Could you check a few things on this drawing? It's one solid part, dimensions in mm from its lowest x, y, z. Coordinates: 2 decimals unless noted, no trailing zeros. Write each loop counter-clockwise with the first axis right and the second up, starting at its lowest first coordinate (ties: lowest second). Pieces come first, ordered by that corner, then holes. Notation, with made-up numbers: M 85,35.5 L 138,35.5 A35 cw 138,72.5 Z; hole C 49,30.25 d1. An arc over 180 degrees is marked long. Use a Markdown table: item, result.
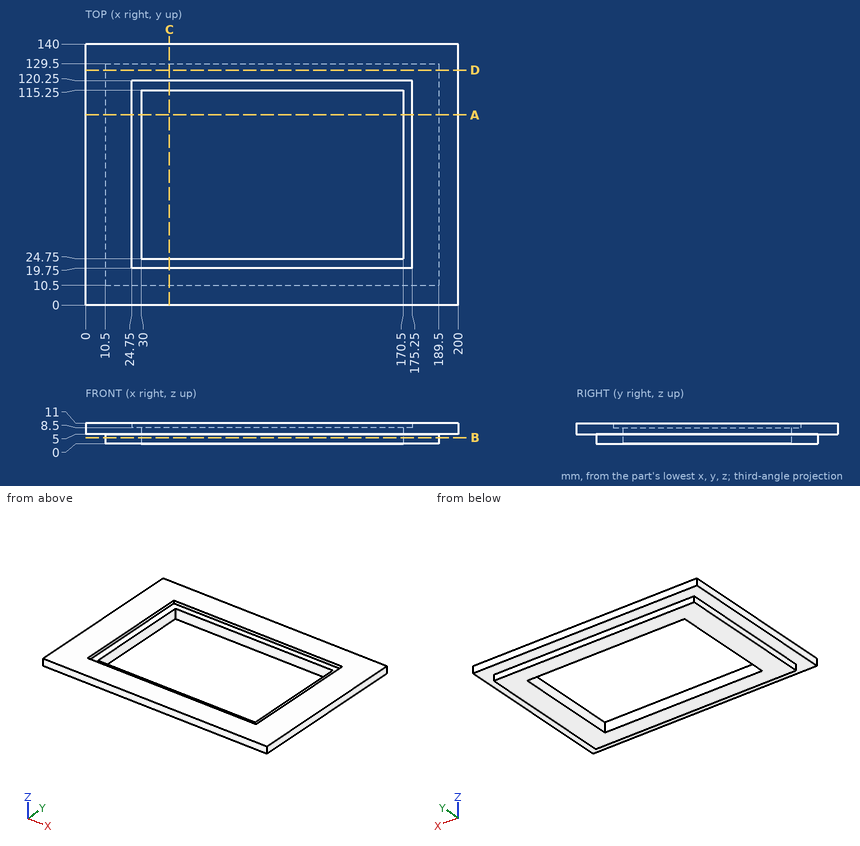
1. Suppose I cut it at C-C on x = 45. Write out the boundary of the cut face in (y, z).
Answers follow:
| item | result |
|---|---|
| outline | M 0,5 L 10.5,5 L 10.5,0 L 24.75,0 L 24.75,8.5 L 19.75,8.5 L 19.75,11 L 0,11 Z; M 115.25,0 L 129.5,0 L 129.5,5 L 140,5 L 140,11 L 120.25,11 L 120.25,8.5 L 115.25,8.5 Z |
2. I need wall thicknesses on probe 1 along X at (y, z) = (114.5, 6.25); probe 2 along Y at (x, z) = (59, 6); probe 3 along X at (y, z) = (95, 10.5). Which ranges of each line are inside material? Lowest first, please.
Answers follow:
| item | result |
|---|---|
| probe 1 | x = 0 to 30, 170.5 to 200 |
| probe 2 | y = 0 to 24.75, 115.25 to 140 |
| probe 3 | x = 0 to 24.75, 175.25 to 200 |
3. Suppose I cut it at D-D on y = 126. Write out the boundary of the cut face in (x, z), and give its area (4 significant figures).
Answers follow:
| item | result |
|---|---|
| outline | M 0,5 L 10.5,5 L 10.5,0 L 189.5,0 L 189.5,5 L 200,5 L 200,11 L 0,11 Z |
| area | 2,095 mm2 |
4. Suppose I cut it at B-B on z = 3.25. Write out the boundary of the cut face in (x, y), and give its area (3 significant figures).
Answers follow:
| item | result |
|---|---|
| outline | M 10.5,10.5 L 189.5,10.5 L 189.5,129.5 L 10.5,129.5 Z; hole M 30,24.75 L 170.5,24.75 L 170.5,115.25 L 30,115.25 Z |
| area | 8,590 mm2 |
5. Will these pins go through, and if not, where does the flat tip stop? pin 1 Ø1.5 at (y, z) = (51, 2) entering from -X; pin 2 Ø5.5 at (x, z) = (109, 1.5) entering from +Y; pin 3 Ø2.5 at (y, z) = (91.5, 3) entering from +X.
Answers follow:
| item | result |
|---|---|
| pin 1 | stops at x = 10.5 |
| pin 2 | stops at y = 129.5 |
| pin 3 | stops at x = 189.5 |
6. Suppose I cut it at A-A on y = 102. Write out the boundary of the cut face in (x, z).
Answers follow:
| item | result |
|---|---|
| outline | M 0,5 L 10.5,5 L 10.5,0 L 30,0 L 30,8.5 L 24.75,8.5 L 24.75,11 L 0,11 Z; M 170.5,0 L 189.5,0 L 189.5,5 L 200,5 L 200,11 L 175.25,11 L 175.25,8.5 L 170.5,8.5 Z |
